Job drawing, mm, ordinate dimensions from the low corner. One solid piece. Give positions to 0.01 mm unless a question says otherwise; leave off trailing zeros. Order: outer loops, then holes, each group sorted by start corner. A loop starts at its lowest first (then second) coordinate and runs counter-clockwise, first axis right, second up. Notation, with made-up numbers: M 69,56 L 128,56 A27 ccw 128,73 Z; hole C -10,41.5 d7. An arc over 180 degrees is marked long. Put each result on its own line as item: value. Start each with the question number.
1) Cut at D-D (z = 23.5). Write the cut outline in (x, y).
2) Cut at A-A (z = 61). Write the cut outline in (x, y).
3) Drill centre lines: line 1 (Y direction, x = 15, z = 45.5); line 2 (X direction, y = 20.5, z = 58) (1 decimal); line 3 (Y direction, x = 17.25, z = 25.5) (1 decimal). Where is each one in solid material? Low to high. Write a range as [from, to].
4) Two-plate mould, pull along Y, no slides. Class the marked faces 1, 2 and 3: released by +Y, released by -Y, zero draft, split by the parting line, or undercut.
5) Cut at C-C (x = 11.25). Write the cut outline in (y, z).
6) Cut at B-B (y = 15). Write the cut outline in (x, z).
7) Pin check, flat tips, straight feed: pin 1 (8 mm diameter, centred on x = 13, z = 46.5, fed in from +Y); pin 2 (1 mm diameter, centred on y = 6.5, z = 13, fed in from -X); pin 3 (2 mm diameter, centred on y = 8.5, z = 9, fed in from +X) (1 decimal); pin 4 (10 mm diameter, centred on y = 7, z = 13.5, fed in from -X). Stop position of each tip, or through.
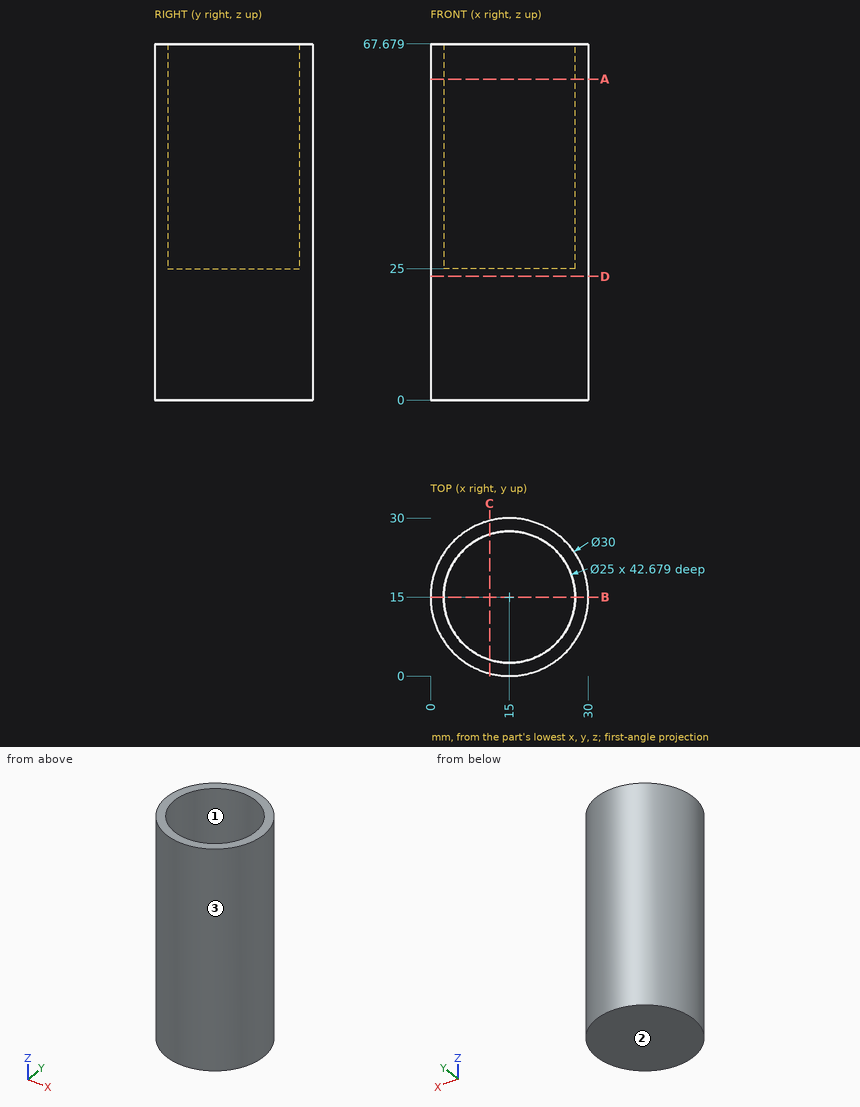
Solution:
1. outline: C 15,15 d30
2. outline: C 15,15 d30; hole C 15,15 d25
3. line 1: [0, 2.5], [27.5, 30]
3. line 2: [1, 3.8], [26.2, 29]
3. line 3: [0.2, 2.7], [27.3, 29.8]
4. face 1: undercut
4. face 2: zero draft
4. face 3: split by the parting line
5. outline: M 0.48,0 L 29.52,0 L 29.52,67.68 L 26.92,67.68 L 26.92,25 L 3.08,25 L 3.08,67.68 L 0.48,67.68 Z
6. outline: M 0,0 L 30,0 L 30,67.68 L 27.5,67.68 L 27.5,25 L 2.5,25 L 2.5,67.68 L 0,67.68 Z
7. pin 1: y = 30
7. pin 2: x = 2.31
7. pin 3: x = 29
7. pin 4: x = 0.3
